Part print with two shaded views. Sizes in mm from the minimum x, y, z corner. A direction names the side the tool comes from. Round coordinates to 2 decimals unless told otherwise and drop trailing zeros. Order: outer loops, then holes, each group sorted by start corner. A loop starts at its lowest first (then second) coordinate and runs counter-clockwise, first axis right, second up. Notation, with made-up numbers: (54.25, -9) -> (87.25, -9) arc R11 ccw to (87.25, -3) -> close; hole circle Ø6 at (-5, 71). An arc over 180 degrees is marked (long way). Use a Markdown table: item, result. Add a question column.
Item 1: Slice it at B-B, the plane z = 10. Give the cut face in (x, y).
Item 2: Probe L1, parallel to Z at x = 53.5, y = 5.25; L2, parallel to X at y = 1.5, z = 25; L3, parallel to X at y = 1.5, z = 10.5. List the from-to ranges inside material, lowest first.
Item 3: Slice it at C-C, the plane x = 28. Give the cut face in (y, z).
Item 4: 3-axis set-ups, long thin cutter, end or side, ignore diameter. For the marked faces 1, 2, 3, 4 and 5: which of +Z, -Z, +X, -X, +Y, -Y reach the whole face in a straight line?
Item 5: Slice it at A-A, the plane y = 5. Give the cut face in (x, z).
Item 6: Pin check, flat tips, straight feed: pin 1 (2 mm diameter, centred on y = 7, z = 20, fed in from -X); pin 2 (3 mm diameter, centred on y = 1.5, z = 43.5, fed in from +X); pin 3 (1.5 mm diameter, centred on x = 8, y = 3.5, fed in from +Z). Stop position of each tip, or through.
Item 7: Slice it at D-D, the plane y = 1.25. Give the cut face in (x, z), plus the area to 3 significant figures.
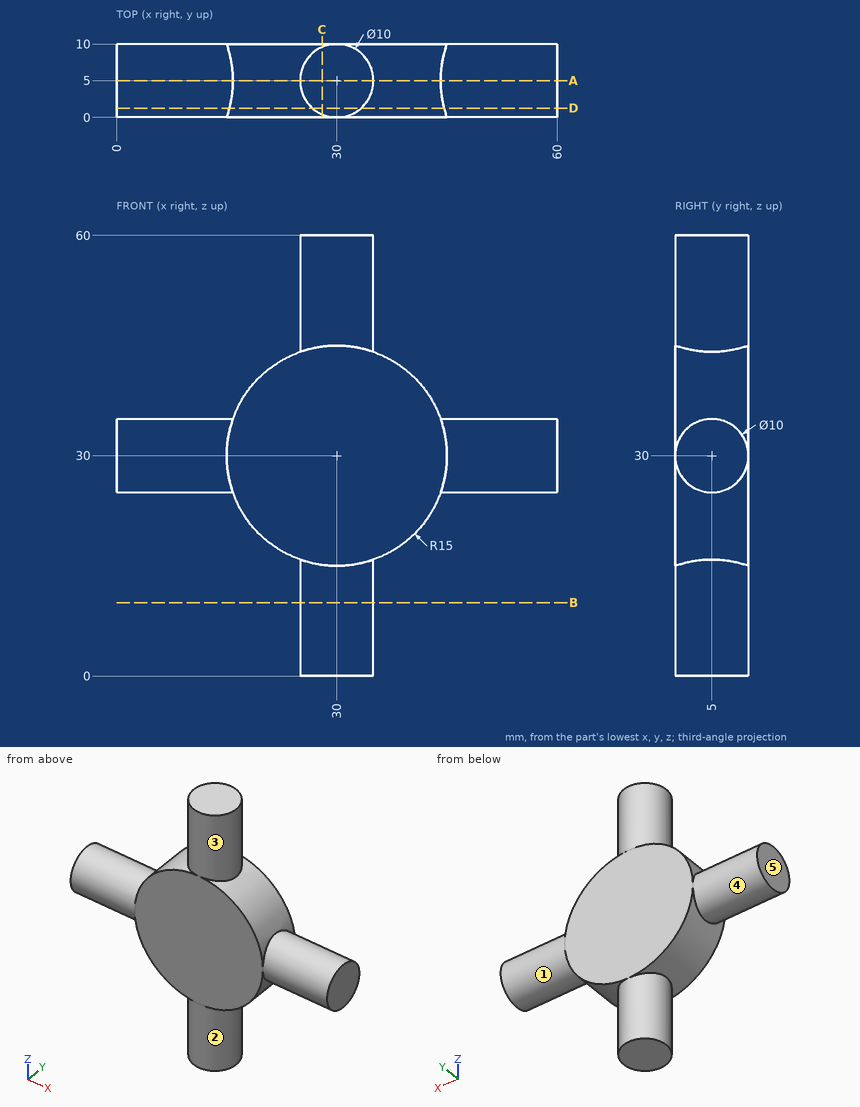
Check sheet entries:
| question | item | result |
|---|---|---|
| 1 | outline | circle Ø10 at (30, 5) |
| 2 | L1 | 25.01 to 34.99 |
| 2 | L2 | 15.86 to 44.14 |
| 2 | L3 | 26.43 to 33.57 |
| 3 | outline | (0, 15.13) -> (0.42, 15.13) -> (0.42, 0) -> (9.58, 0) -> (9.58, 15.13) -> (10, 15.13) -> (10, 44.87) -> (9.58, 44.87) -> (9.58, 60) -> (0.42, 60) -> (0.42, 44.87) -> (0, 44.87) -> close |
| 4 | face 1 | +X |
| 4 | face 2 | -Z |
| 4 | face 3 | +Z |
| 4 | face 4 | -X |
| 4 | face 5 | +Z, -Z, -X, +Y, -Y |
| 5 | outline | (0, 25) -> (15.86, 25) arc R15 ccw to (25, 15.86) -> (25, 0) -> (35, 0) -> (35, 15.86) arc R15 ccw to (44.14, 25) -> (60, 25) -> (60, 35) -> (44.14, 35) arc R15 ccw to (35, 44.14) -> (35, 60) -> (25, 60) -> (25, 44.14) arc R15 ccw to (15.86, 35) -> (0, 35) -> close |
| 6 | pin 1 | x = 18 |
| 6 | pin 2 | x = 39 |
| 6 | pin 3 | z = 34.94 |
| 7 | outline | (0, 26.69) -> (15.37, 26.69) arc R15 ccw to (26.69, 15.37) -> (26.69, 0) -> (33.31, 0) -> (33.31, 15.37) arc R15 ccw to (44.63, 26.69) -> (60, 26.69) -> (60, 33.31) -> (44.63, 33.31) arc R15 ccw to (33.31, 44.63) -> (33.31, 60) -> (26.69, 60) -> (26.69, 44.63) arc R15 ccw to (15.37, 33.31) -> (0, 33.31) -> close |
| 7 | area | 1,110 mm2 |
